```python
from build123d import *

# Parameters (mm, degrees)
SALIENTE_EXTRUIR1_DEPTH = 37.5285
CORTAR_EXTRUIR1_DEPTH   = 18.4023
SALIENTE_EXTRUIR2_DEPTH = 15.0114
SALIENTE_EXTRUIR3_DEPTH = 53.975
CORTAR_EXTRUIR2_DEPTH   = 17.1323
CROQUIS6_W              = 24.9936
CROQUIS6_H              = 37.5285
CROQUIS6_W_2            = 2.54
CROQUIS6_H_2            = 27.79
SALIENTE_EXTRUIR4_DEPTH = 2.54
SALIENTE_EXTRUIR5_DEPTH = 1.9939
SALIENTE_EXTRUIR6_DEPTH = 17.1323
SALIENTE_EXTRUIR7_DEPTH = 18.683041561
SALIENTE_EXTRUIR8_DEPTH = 19.015985732
SALIENTE_EXTRUIR9_DEPTH = 17.1323
CHAFL_N1_SIZE           = 2.54


with BuildPart() as part:
    # Croquis1 → Saliente-Extruir1 (new body)
    with BuildSketch(Plane(origin=(0, 19.7612, 0), x_dir=(1, 0, 0), z_dir=(0, 1, 0))):
        Polygon((0, 12.4968), (24.9936, -12.4968), (24.9936, 12.4968), align=None)
    extrude(amount=-SALIENTE_EXTRUIR1_DEPTH)

    # Croquis2 → Cortar-Extruir1 (cut)
    with BuildSketch(Plane.XZ.offset(17.7673)):
        Polygon((24.9936, -10.5029), (24.9936, 10.5029), (22.9997, 10.5029), (1.9939, -10.5029), align=None)
    extrude(amount=-CORTAR_EXTRUIR1_DEPTH, mode=Mode.SUBTRACT)

    # Croquis3 → Saliente-Extruir2 (add)
    with BuildSketch(Plane(origin=(24.9936, 0, 0), x_dir=(0, 0, -1), z_dir=(1, 0, 0))):
        Polygon((10.5029, -17.7673), (10.5029, 0.635), (-10.5029, 0.635), (-10.5029, -17.7673), (-12.4968, -17.7673), (-12.4968, 19.7612), (12.4968, 19.7612), (12.4968, -17.7673), align=None)
    extrude(amount=SALIENTE_EXTRUIR2_DEPTH)

    # Croquis4 → Saliente-Extruir3 (add)
    with BuildSketch(Plane(origin=(40.005, 0, 0), x_dir=(0, 0, -1), z_dir=(1, 0, 0))):
        Polygon((10.5029, 1.469986946), (-10.5029, 1.469986946), (-10.5029, -17.7673), (-12.4968, -17.7673), (-12.4968, 19.7612), (12.4968, 19.7612), (12.4968, -17.7673), (10.5029, -17.7673), align=None)
    extrude(amount=SALIENTE_EXTRUIR3_DEPTH)

    # Croquis5 → Cortar-Extruir2 (cut)
    with BuildSketch(Plane.XZ.offset(-0.635)):
        Polygon((93.98, -10.5029), (93.98, 10.5029), (22.9997, 10.5029), (1.9939, -10.5029), align=None)
    extrude(amount=-CORTAR_EXTRUIR2_DEPTH, mode=Mode.SUBTRACT)

    # Croquis6 → Saliente-Extruir4 (add)
    with BuildSketch(Plane(origin=(93.98, 0, 0), x_dir=(0, 0, -1), z_dir=(1, 0, 0))):
        with Locations((0, 0.99695)):
            Rectangle(CROQUIS6_W, CROQUIS6_H)
        with Locations((0, 0.0012)):
            Rectangle(CROQUIS6_W_2, CROQUIS6_H_2, mode=Mode.SUBTRACT)
    extrude(amount=SALIENTE_EXTRUIR4_DEPTH)

    # Croquis7 → Saliente-Extruir5 (add)
    with BuildSketch(Plane.XZ.offset(17.7673)):
        Polygon((24.9936, 12.4968), (96.52, 12.4968), (96.52, -12.4968), (0, -12.4968), align=None)
    extrude(amount=SALIENTE_EXTRUIR5_DEPTH)

    # Croquis8 → Saliente-Extruir6 (add)
    with BuildSketch(Plane(origin=(0, -17.7673, 0), x_dir=(-1, 0, 0), z_dir=(0, 1, 0))):
        Polygon((-65.405, -4.138152009), (-65.405, -10.5029), (-68.58, -10.5029), (-68.58, -3.819468452), align=None)
    extrude(amount=SALIENTE_EXTRUIR6_DEPTH)

    # Croquis9 → Saliente-Extruir7 (add)
    with BuildSketch(Plane.XZ.offset(-17.7673)):
        Polygon((65.405, 10.5029), (68.58, 10.5029), (68.58, 4.573954196), (65.405, 4.98694847), align=None)
    extrude(amount=SALIENTE_EXTRUIR7_DEPTH)

    # Croquis10 → Saliente-Extruir8 (add)
    with BuildSketch(Plane.XZ.offset(-17.7673)):
        Polygon((68.58, -3.819468452), (68.58, -10.5029), (65.405, -10.5029), (65.405, -4.138152009), align=None)
    extrude(amount=SALIENTE_EXTRUIR8_DEPTH)

    # Croquis11 → Saliente-Extruir9 (add)
    with BuildSketch(Plane(origin=(0, -17.7673, 0), x_dir=(-1, 0, 0), z_dir=(0, 1, 0))):
        Polygon((-68.58, 10.5029), (-65.405, 10.5029), (-65.405, 4.98694847), (-68.58, 4.573954196), align=None)
    extrude(amount=SALIENTE_EXTRUIR9_DEPTH)

    # Chaflán1
    chafl_n1_edges = [part.edges().sort_by_distance(p)[0] for p in [
        (81.28, -17.7673, -10.5029),
        (44.20235, 17.7673, 10.5029),
        (81.28, 17.7673, -10.5029),
        (33.69945, -17.7673, -10.5029),
        (81.28, -17.7673, 10.5029),
        (44.20235, -17.7673, 10.5029),
        (33.69945, 17.7673, -10.5029),
        (81.28, 17.7673, 10.5029),
    ]]
    chamfer(chafl_n1_edges, length=CHAFL_N1_SIZE)


solid = part.part
```
Read the model definition and answer for the solid it produces. Units are mm, in the model's axes. A direction names the side the tool comes from. Round coordinates to 2 decimals unless told otherwise and drop trailing zeros. Write each loop counter-clockwise with the first axis right and the second up, starting at its lowest first coordinate (ties: lowest second). Pieces come first, ordered by that corner, then holes. Notation, with made-up numbers: (28.5, 41.25) -> (38.5, 41.25) arc R22 cw to (38.5, 68.25) -> close; hole circle Ø3 at (-1.75, -38). An arc over 180 degrees is marked (long way). Answer in a Markdown table with one row per item. Add a question column.
1) Find section D-D, the plane z = -6. Determine the outline of the cut face in (x, y) (3 decimals), and give its area (3 significant figures).
2) Given P1, Ø10, axis at y = 9, z = -0.5, coming from the -X side (3 decimals), flat-ended and moving along its own axis, determine where the tip first touches the part or whether it passes through.
3) Which of the six approach directions +Z, -Z, +X, -X, +Y, -Y give full straight-line access (tool end or side, diameter ignored) to faces 4 (the face through (65.405, 0, 8)), 5 (the face through (81.458, 16.515, 9.215)), 6 (the face through (95, -13.894, 0)), 7 (the face through (49, 0, -12.497))?
4) Find section C-C, the plane x = 55.5. Determine the outline of the cut face in (y, z).
5) Find section B-B, the plane y = 5. Determine the outline of the cut face in (x, z) (3 decimals), and give its area (3 significant figures).
6) Determine the mould class of faces 1 (the face through (60, -19.761, 0)), 2 (the face through (1.33, 1.556, -11.167)), 3 (the face through (95, 0, -1.27)) for opening direction Y: pulls with the +Y half, pulls with the -Y half, needs draft (parallel to the pull), parting line crosses it, or undercut.
7) Find section A-A, the plane z = 0. Determine the outline of the cut face in (x, y), and give its area (3 significant figures).
8) Consider line 1 (X direction, y = -16, z = -4.75) (3 decimals); line 2 (Y direction, x = 72, z = 4); line 3 (Z direction, x = 44.5, y = 10). Determine where each line is inside the solid, lowest interval first.
Findings below:
| question | item | result |
|---|---|---|
| 1 | outline | (6.497, -19.761) -> (96.52, -19.761) -> (96.52, 19.761) -> (6.497, 19.761) -> (6.497, 17.767) -> (65.405, 17.767) -> (65.405, -17.767) -> (6.497, -17.767) -> close; hole (68.58, -17.767) -> (93.98, -17.767) -> (93.98, 17.767) -> (68.58, 17.767) -> close |
| 1 | area | 562 mm² |
| 2 | P1 | x = 65.405 |
| 3 | face 4 | -X |
| 3 | face 5 | none |
| 3 | face 6 | +X, -X |
| 3 | face 7 | -Z, +X, -X, +Y, -Y |
| 4 | outline | (-19.76, -12.5) -> (19.76, -12.5) -> (19.76, 12.5) -> (-19.76, 12.5) -> close; hole (-17.77, -7.96) -> (-15.23, -10.5) -> (15.23, -10.5) -> (17.77, -7.96) -> (17.77, 7.96) -> (15.23, 10.5) -> (-15.23, 10.5) -> (-17.77, 7.96) -> close |
| 5 | outline | (0, -12.497) -> (96.52, -12.497) -> (96.52, -1.27) -> (93.98, -1.27) -> (93.98, -10.503) -> (68.58, -10.503) -> (68.58, -3.819) -> (65.405, -4.138) -> (65.405, -10.503) -> (1.994, -10.503) -> close; (23, 10.503) -> (65.405, 10.503) -> (65.405, 4.987) -> (68.58, 4.574) -> (68.58, 10.503) -> (93.98, 10.503) -> (93.98, 1.27) -> (96.52, 1.27) -> (96.52, 12.497) -> (24.994, 12.497) -> close |
| 5 | area | 421 mm² |
| 6 | face 1 | pulls with the -Y half |
| 6 | face 2 | needs draft |
| 6 | face 3 | undercut |
| 7 | outline | (12.5, -19.76) -> (96.52, -19.76) -> (96.52, -13.89) -> (93.98, -13.89) -> (93.98, -17.77) -> (12.5, -17.77) -> close; (12.5, 17.77) -> (93.98, 17.77) -> (93.98, 13.9) -> (96.52, 13.9) -> (96.52, 19.76) -> (12.5, 19.76) -> close |
| 7 | area | 355 mm² |
| 8 | line 1 | 65.405 to 68.58, 93.98 to 96.52 |
| 8 | line 2 | -19.76 to -17.77, 17.77 to 19.76 |
| 8 | line 3 | -12.5 to -10.5, 10.5 to 12.5 |
